Source: CAD feature listing. Evaluate the final solid. Frame: model axes, mm. A direction names the side the tool comes from. Give positions to 0.01 mm unless a question says otherwise; leave off trailing zeros. Write each loop counter-clockwise with the first axis right and the second up, starting at its lowest first coordinate (ties: lowest second). Pieces come first, ordered by that corner, then holes. Notation, with made-up numbers: M 72,59 L 124,59 A16 cw 124,63 Z; hole C 7,-27.5 d3. An arc over 180 degrees is marked long. Return JSON: item names as keys, results as strings.
Autodesk Inventor part; units mm, degrees
ref_plane "Work Plane1" through (0, -862.1118, 0) normal (0, 0, 1) x (-1, 0, 0)
ref_plane "YZ Plane" through (0, 0, 0) normal (1, 0, 0) x (0, 1, 0)
ref_plane "XZ Plane" through (0, 0, 0) normal (0, 1, 0) x (-1, 0, 0)
ref_plane "Work Plane1" through (0, -862.1118, 0) normal (0, 0, 1) x (-1, 0, 0)
sketch "Sketch1" plane through (0, -862.1118, 0) normal (0, 0, 1) x (-1, 0, 0)
  circle A0 centre (-188, -18) radius 4 construction
  line L0 (-220, -478) -> (-220, 22) construction
  line L1 (-220, -478) -> (-208, -478) construction
  line L2 (-208, 22) -> (-208, -478) construction
  line L3 (-220, 22) -> (-208, 22) construction
  line L4 (-208, -29.2209) -> (-198, -29.2209)
  line L5 (-198, -109.2209) -> (-208, -109.2209)
  line L6 (-208, -109.2209) -> (-208, -29.2209)
  line L7 (-158, -47.7209) -> (-198, -47.7209)
  line L8 (-198, -90.7209) -> (-158, -90.7209)
  line L9 (-158, -90.7209) -> (-158, -47.7209)
  circle A1 centre (-179.15, -68.8709) radius 11.5
  circle A2 centre (-164, -53.7209) radius 2
  circle A3 centre (-195, -53.7209) radius 2
  circle A4 centre (-195, -84.7209) radius 2
  circle A5 centre (-164, -84.7209) radius 2
  line L10 (-195, -84.7209) -> (-195, -53.7209) construction
  line L11 (-195, -84.7209) -> (-164, -84.7209) construction
  line L12 (-198, -29.2209) -> (-198, -47.7209)
  line L13 (-198, -90.7209) -> (-198, -109.2209)
  point P0 (0, -862.1118)
  dimension "d0" = 10
  dimension "d1" = 80
  dimension "d3" = 43
  dimension "d4" = 18.5
  dimension "d5" = 18.5
  dimension "d6" = 23
  dimension "d7" = 4
  dimension "d8" = 4
  dimension "d9" = 4
  dimension "d10" = 4
  dimension "d11" = 31
  dimension "d12" = 31
  dimension "d13" = 31
  dimension "d14" = 31
  dimension "d15" = 6
  dimension "d18" = 6
  dimension "d19" = 6
  dimension "d20" = 6
  dimension "d21" = 90
  dimension "d25" = 21.15
  dimension "d26" = 21.15
  dimension "d27" = 90
  dimension "d28" = 90
  dimension "d29" = 18.5
  dimension "d41" = 40
  dimension "d42" = 40
extrude "Tykkelse" add sketch "Sketch1" along normal blind 10
sketch "Sketch2" plane through (198, -832.8909, 0) normal (-1, 0, 0) x (0, 0, 1)
  line L0 (0, 0) -> (10, 0)
  line L1 (10, 18.5) -> (10, 0)
  line L2 (0, 80) -> (0, 61.5)
  line L3 (0, 61.5) -> (10, 61.5)
  line L4 (10, 80) -> (10, 61.5)
  line L5 (0, 80) -> (10, 80)
  circle A0 centre (5, 70) radius 2.5
  circle A1 centre (5, 10) radius 2.5
  point P0 (0, 832.8909)
  dimension "d32" = 5
  dimension "d33" = 5
  dimension "d34" = 10
  dimension "d35" = 5
  dimension "d36" = 5
  dimension "d37" = 10
extrude "Befæstelseshuller" cut sketch "Sketch2" against normal up to surface (10 mm away) contours A0 | A1
fillet "Fillet1" radius 0.5 8 edges at (198, -814.3909, 5) (198, -771.3909, 5) (158, -771.3909, 5) (158, -814.3909, 5) (198, -832.8909, 5) (208, -832.8909, 5) (198, -752.8909, 5) (208, -752.8909, 5)
equation "\"d4\" = d5"
equation "\"d8\" = d7"
equation "\"d9\" = d7"
equation "\"d10\" = d7"
equation "\"d13\" = d11"
equation "\"d14\" = d12"
equation "\"d15\" = d20"
equation "\"d18\" = d15"
equation "\"d19\" = d18"
equation "\"d42\" = d41"
equation "\"d32\" = d33"
equation "\"d36\" = d35"
equation "\"d37\" = d34"
properties part number "Stepper Holder X&Y_3" material "Aluminum 6061"
1) Contact query for flat-ended pins moving along their axis: pin 1 Ø3 at (x, z) = (175, 4) entering from -Y; pin 2 Ø4 at (x, z) = (193.5, 2) entering from +Y; pin 3 Ø5 at (y, z) = (-762, 6) entering from -X. Output: stop coordinate, or through.
Numbers:
{"pin 1": "stops at y = -814.39", "pin 2": "stops at y = -771.39", "pin 3": "stops at x = 198"}
2) Cut plane B-B, the plane z = 5. Give the number of separate pieces and of enclosed holes in the cut face, then the cut area to 3 significant figures.
Numbers:
{"separate pieces": "3", "enclosed holes": "5", "area": "1,950 mm²"}
3) Set-up query: faces 1 (the face through (198, -826, 5)), 2 (the face through (194, -793, 10)), 3 (the face through (198, -760, 5)). Return all of +Z, -Z, +X, -X, +Y, -Y with unobstructed straight access to the full face (end or side cutting, diameter ignored); none if empty.
Numbers:
{"face 1": "+Z, -Z, -X, -Y", "face 2": "+Z, +X, -X, +Y, -Y", "face 3": "+Z, -Z, -X, +Y"}
4) Cut plane D-D, the plane x = 179.15. Return the cut outline in (y, z).
Numbers:
{"outline": "M -814.39,0 L -804.74,0 L -804.74,10 L -814.39,10 Z; M -781.74,0 L -771.39,0 L -771.39,10 L -781.74,10 Z"}
5) Draft query along Z for faces 4 (the face through (202.93, -825.33, 4.46)), 5 (the face through (194, -793, 0)), 6 (the face through (203, -832.891, 5)). Return one class per face: released by +Z, released by -Z, zero draft, split by the parting line, or undercut.
Numbers:
{"face 4": "undercut", "face 5": "released by -Z", "face 6": "zero draft"}
6) Cut plane C-C, the plane y = -788. Return the cut outline in (x, z).
Numbers:
{"outline": "M 158,0 L 168.91,0 L 168.91,10 L 158,10 Z; M 189.39,0 L 208,0 L 208,10 L 189.39,10 Z"}
7) Cut plane A-A, the plane x = 164. Return the cut outline in (y, z), then the cut area to 3 significant figures.
Numbers:
{"outline": "M -814.39,0 L -810.39,0 L -810.39,10 L -814.39,10 Z; M -806.39,0 L -779.39,0 L -779.39,10 L -806.39,10 Z; M -775.39,0 L -771.39,0 L -771.39,10 L -775.39,10 Z", "area": "350 mm²"}
8) Line query: line 1 (Y direction, x = 195, z = 7.5); line 2 (Y direction, x = 205.5, z = 5); line 3 (X direction, y = -776, z = 3). Output: solid intervals per line, ascending. Write a range as [from, to].
Numbers:
{"line 1": "y = [-814.39, -810.39], [-806.39, -779.39], [-775.39, -771.39]", "line 2": "y = [-832.89, -825.39], [-820.39, -765.39], [-760.39, -752.89]", "line 3": "x = [158, 162.56], [165.44, 193.56], [196.44, 208]"}
